from build123d import *

# Parameters (mm, degrees)
F0_W     = 127
F0_H     = 44.45
F1_DEPTH = 609.6
F2_R     = 6.35
F3_T     = 6.35


# Not quite as in the source:
# - a shell that OpenCascade refuses in one call is made with other operations: the cavity is built on its own and cut out


with BuildPart() as f1:
    # F0 (on Right) → F1 (new body, symmetric)
    with BuildSketch(Plane.YZ):
        with Locations((0, -22.225)):
            Rectangle(F0_W, F0_H)
    extrude(amount=F1_DEPTH, both=True)

    # F2
    f2_edges = [f1.edges().sort_by_distance(p)[0] for p in [
        (0, -63.5, 0),
        (0, 63.5, 0),
    ]]
    fillet(f2_edges, radius=F2_R)

    # F3: shell of thickness 6.35, made by hand


with BuildPart() as f3_core1:
    # F3_t2: copy of F1
    add(f1.part)

    # the walls: a layer under each face that stays
    f3_faces = [f3_core1.faces().sort_by_distance(p)[0] for p in [
        (0, 0, 0),
        (0, 63.5, -25.4),
        (0, -63.5, -25.4),
    ]]
    thicken(f3_faces, amount=-F3_T, mode=Mode.SUBTRACT)


with BuildPart() as f1_1:
    add(f1.part)

    # what is left inside the walls is the cavity
    f3_cavity = [f3_core1.part.solids().sort_by_distance(p)[0] for p in [
        (-203.2, 0, -44.3865),
    ]]
    add(f3_cavity, mode=Mode.SUBTRACT)


solid = f1_1.part
Input: part model. Units: mm. Frame: model coordinates. A direction names the side the tool comes from. Coordinates: 2 decimals unless noted, no trailing zeros. Loops run counter-clockwise (first coordinate to the right, second up) from the corner with the lowest first, then second, coordinate; pieces in that order, holes last.
(1) Section A-A on z = -33. Return the cut outline in (x, y).
(2) Set-up query: faces 1 (the face through (-609.6, 0, -6)), 2 (the face through (9, 57.15, -26)). Return all of +Z, -Z, +X, -X, +Y, -Y with unobstructed straight access to the full face (end or side cutting, diameter ignored); none if empty.
(3) Material intervals for probe 1 along Y at (x, z) = (-424.5, -36); probe 2 along Z at (x, y) = (117.5, -50.5); probe 3 along Y at (x, z) = (-133, -5), sorted ascending.
(4) Pull-direction query (Y, two-part tool) for faces 3 (the face through (9, -63.5, -26)), 4 (the face through (9, 63.5, -26)), 5 (the face through (9, -57.15, -26)); classes: released by +Y, released by -Y, zero draft, split by the parting line, or undercut.
(5) Section C-C on y = 23.5. Return the cut outline in (x, z), then the cut area to 3 significant figures.
(6) Section B-B on x = 479. Return the cut outline in (y, z), then the cut area to 3 significant figures.
Data:
1. outline: (-609.6, -63.5) - (609.6, -63.5) - (609.6, -57.15) - (-609.6, -57.15) - close; (-609.6, 57.15) - (609.6, 57.15) - (609.6, 63.5) - (-609.6, 63.5) - close
2. face 1: +Z, -Z, -X, +Y, -Y
2. face 2: -Z, +X, -X
3. probe 1: y = -63.5 to -57.15, 57.15 to 63.5
3. probe 2: z = -6.35 to 0
3. probe 3: y = -63.35 to 63.35
4. face 3: released by -Y
4. face 4: released by +Y
4. face 5: undercut
5. outline: (-609.6, -6.35) - (609.6, -6.35) - (609.6, 0) - (-609.6, 0) - close
5. area: 7,740 mm2
6. outline: (-63.5, -44.45) - (-57.15, -44.45) - (-57.15, -6.35) - (57.15, -6.35) - (57.15, -44.45) - (63.5, -44.45) - (63.5, -6.35) arc R6.35 ccw to (57.15, 0) - (-57.15, 0) arc R6.35 ccw to (-63.5, -6.35) - close
6. area: 1,270 mm2
